Answer from the drawing. Dimensions are ordinates in mm from the lowest x, y and z of the part. Coordinates: 2 decimals unless noted, no trailing zeros. Write each loop counter-clockwise with the first axis right and the second up, starting at its lowest first coordinate (ties: lowest second). Pieces come first, ordered by that corner, then holes. Notation, with made-up numbers: (64, 34.5) - (100, 34.5) arc R13 cw to (100, 54.5) - close; hole circle Ø11 at (39, -2). An arc over 180 degrees is marked (long way). Answer as a JSON object with one key per item and string values. Group by question number.
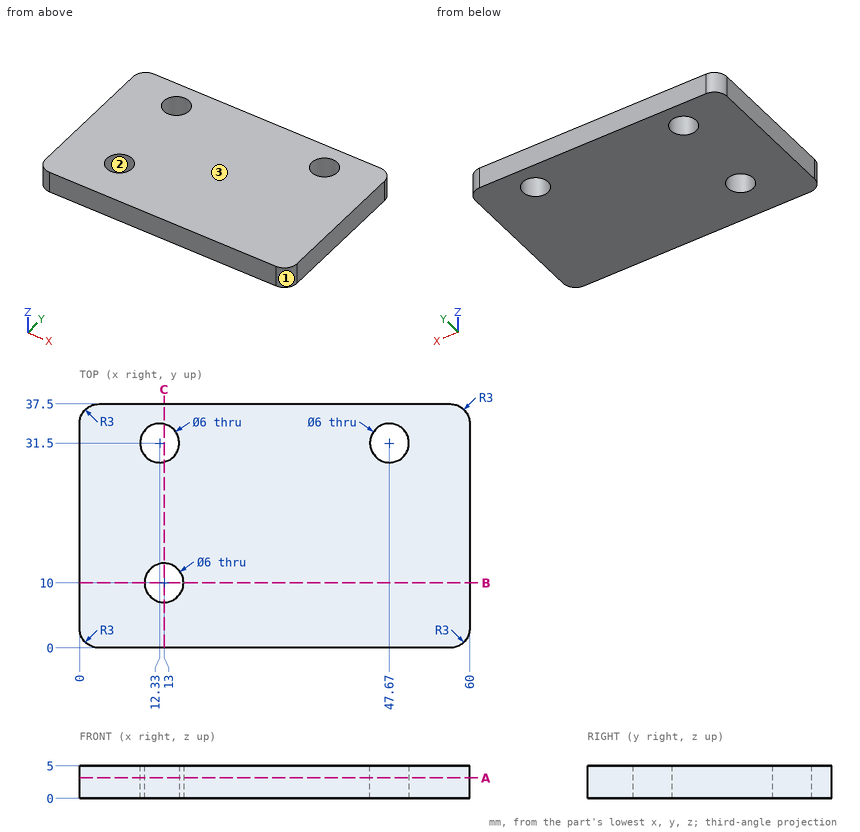
Q1. Section C-C on x = 13 is taken. Determine the outline of the cut face in (y, z).
Q2. Consider L1, parallel to X at y = 32.5, z = 0.6; L2, parallel to Y at x = 12.33, z = 1.8; L3, parallel to Y at x = 13, z = 2.3. Determine where each line is inside the solid, lowest interval first. Write a range as from..to.
Q3. A flat-ended cylindrical pin translates along its axis: pin 1 Ø5.5 at (x, y) = (12.33, 31.5) entering from -Z. Find the tip coordinate at first contact, or state that the pin passes through.
Q4. Section B-B on y = 10 is taken. Determine the outline of the cut face in (x, z).
Q5. Section A-A on z = 3.15 is taken. Determine the outline of the cut face in (x, y).
Q6. For a pull along Y with two mould halves and no side action, classify the marked faces 1, 2 and 3 as +Y half, -Y half, draft (parallel to the pull), parting line (faces both ways), or undercut.
Numbers:
{
 "1": {"outline": "(0, 0) - (7, 0) - (7, 5) - (0, 5) - close; (13, 0) - (28.58, 0) - (28.58, 5) - (13, 5) - close; (34.42, 0) - (37.5, 0) - (37.5, 5) - (34.42, 5) - close"},
 "2": {"L1": "x = 0..9.5, 15.16..44.84, 50.5..60", "L2": "y = 0..7.08, 12.92..28.5, 34.5..37.5", "L3": "y = 0..7, 13..28.58, 34.42..37.5"},
 "3": {"pin 1": "passes through"},
 "4": {"outline": "(0, 0) - (10, 0) - (10, 5) - (0, 5) - close; (16, 0) - (60, 0) - (60, 5) - (16, 5) - close"},
 "5": {"outline": "(0, 3) arc R3 ccw to (3, 0) - (57, 0) arc R3 ccw to (60, 3) - (60, 34.5) arc R3 ccw to (57, 37.5) - (3, 37.5) arc R3 ccw to (0, 34.5) - close; hole circle Ø6 at (12.33, 31.5); hole circle Ø6 at (13, 10); hole circle Ø6 at (47.67, 31.5)"},
 "6": {"face 1": "-Y half", "face 2": "undercut", "face 3": "draft"}
}
